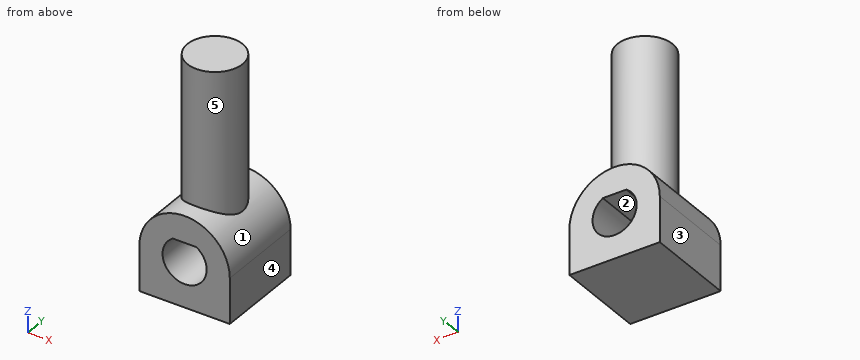
from build123d import *

# Parameters (mm, degrees)
PAD015_DEPTH    = 12.7
SKETCH033_R     = 3.8862
PAD016_DEPTH    = 25.4
POCKET016_DEPTH = 12.701


with BuildPart() as part:
    # Sketch032 → Pad015 (new body)
    with BuildSketch(Plane.XZ):
        with BuildLine():
            ThreePointArc((6.35, 0), (0, 6.35), (-6.35, 0))
            Line((-6.35, 0), (-6.35, -6.35))
            Line((-6.35, -6.35), (6.35, -6.35))
            Line((6.35, -6.35), (6.35, 0))
        make_face()
    extrude(amount=PAD015_DEPTH)

    # Sketch033 (on DatumPlane) → Pad016 (join)
    with BuildSketch(Plane(origin=(0, 0, 0), x_dir=(1, 0, 0), z_dir=(0, 0, -1))):
        with Locations((0, 6.35)):
            Circle(SKETCH033_R)
    extrude(amount=-PAD016_DEPTH)

    # Sketch034 (on Face4 of Pad016) → Pocket016 (cut, through all)
    with BuildSketch(Plane.XZ.offset(12.7)):
        with BuildLine():
            ThreePointArc((-1.651, 2.622358), (0, -3.0988), (1.651, 2.622358))
            Line((-1.651, 2.622358), (1.651, 2.622358))
        make_face()
    extrude(amount=-POCKET016_DEPTH, mode=Mode.SUBTRACT)


solid = part.part
Model file for the job. Use its own axes, mm. Face numbers are marked on the shaded views. A direction names the side the tool comes from. Give positions to 0.01 mm unless a question says otherwise; leave off trailing zeros. Loops run counter-clockwise (first coordinate to the right, second up) from the corner with the lowest first, then second, coordinate; pieces in that order, holes last. Notation, with made-up numbers: (69.5, -33) -> (127.5, -33) arc R15 cw to (127.5, -5) -> close; hole circle Ø1 at (60, 39.5). An arc over 180 degrees is marked (long way). Use a Markdown table: item, result. Add a question column.
(1) Slice it at D-D on x = -2. List the corners of the cut face in (y, z), and give its area (3 significant figures).
(2) Wall check: line 1 along Z through (x, y) = (0, -5.75); line 2 along Z through (x, y) = (-2, -6.25); line 3 along X through (y, z) = (-11.5, -2.5). Give the ranges that are in metal, low to high.
(3) Mould opens along Z. For the marked faces 1, 2 and 3 say: +Z half, -Z half, draft (parallel to the pull), parting line (faces both ways), or undercut.
(4) Tool access for the marked faces 4 and 5: list every direction of +Z, -Z, +X, -X, +Y, -Y with a clear straight run to the whole face (end or side of a thin tool).
(5) Slice it at C-C on y = -6. List the corners of the cut face in (x, z).
(6) Drop flat-ended pins along their axis: pin 1 Ø4 at (y, z) = (-7.5, 11) entering from +X; pin 2 Ø2 at (x, y) = (4, -2) entering from +Z; pin 3 Ø5 at (x, z) = (4, 20) entering from +Y. Give the stop position or say it passes through.
(7) Slice it at B-B on z = -1. List the corners of the cut face in (x, y), and give its area (3 significant figures).
(8) Slice it at A-A on x = 0. List the corners of the cut face in (y, z).
Filled sheet:
| question | item | result |
|---|---|---|
| 1 | outline | (-12.7, -6.35) -> (0, -6.35) -> (0, -2.37) -> (-12.7, -2.37) -> close; (-12.7, 2.37) -> (0, 2.37) -> (0, 6.03) -> (-3.02, 6.03) -> (-3.02, 25.4) -> (-9.68, 25.4) -> (-9.68, 6.03) -> (-12.7, 6.03) -> close |
| 1 | area | 226 mm2 |
| 2 | line 1 | -6.35 to -3.1, 2.62 to 25.4 |
| 2 | line 2 | -6.35 to -2.37, 2.37 to 25.4 |
| 2 | line 3 | -6.35 to -1.83, 1.83 to 6.35 |
| 3 | face 1 | +Z half |
| 3 | face 2 | undercut |
| 3 | face 3 | draft |
| 4 | face 4 | +Z, -Z, +X, +Y, -Y |
| 4 | face 5 | +Z |
| 5 | outline | (-6.35, -6.35) -> (6.35, -6.35) -> (6.35, 0) arc R6.35 ccw to (3.87, 5.03) -> (3.87, 25.4) -> (-3.87, 25.4) -> (-3.87, 5.03) arc R6.35 ccw to (-6.35, 0) -> close; hole (-1.65, 2.62) arc R3.1 ccw (long way) to (1.65, 2.62) -> close |
| 6 | pin 1 | x = 3.89 |
| 6 | pin 2 | z = 5.6 |
| 6 | pin 3 | y = -2.76 |
| 7 | outline | (-6.35, -12.7) -> (-2.93, -12.7) -> (-2.93, 0) -> (-6.35, 0) -> close; (2.93, -12.7) -> (6.35, -12.7) -> (6.35, 0) -> (2.93, 0) -> close |
| 7 | area | 86.8 mm2 |
| 8 | outline | (-12.7, -6.35) -> (0, -6.35) -> (0, -3.1) -> (-12.7, -3.1) -> close; (-12.7, 2.62) -> (0, 2.62) -> (0, 6.35) -> (-2.46, 6.35) -> (-2.46, 25.4) -> (-10.24, 25.4) -> (-10.24, 6.35) -> (-12.7, 6.35) -> close |
